Source: CAD feature listing. Evaluate the final solid. Frame: model axes, mm. A direction names the side the tool comes from. Round coordinates to 2 decimals unless told otherwise and drop trailing zeros. Loops run counter-clockwise (first coordinate to the right, second up) from the corner with the lowest first, then second, coordinate; pieces in that order, holes last. Notation, with made-up numbers: M -26,-35.5 L 28,-35.5 A30 ccw 28,-11.5 Z; hole C 86,-1 d7. An arc over 180 degrees is marked long. Answer as CSV lines item,"result". Start each with the question number.
```python
from build123d import *

# Parameters (mm, degrees)
ESBO_O3_W = 2.1
ESBO_O3_H = 15.4
FILETE1_R = 3
FILETE2_R = 0.5


with BuildPart() as part:
    # Esboço1 → Revolução1 (revolve)
    with BuildSketch(Plane.XY, mode=Mode.PRIVATE) as revolu_o1_sk:
        Polygon((0, 10.8), (0, 15.4), (15, 15.4), (15, 13.5), (50, 13.5), (50, 10.8), align=None)
    revolve(revolu_o1_sk.sketch.rotate(Axis((0, 0, 0), (1, 0, 0)), 90), axis=Axis((0, 0, 0), (1, 0, 0)))

    # Esboço3 → Furo roscado de M51 (revolve, cut)
    with BuildSketch(Plane(origin=(35, 0, 0), x_dir=(0, 0, -1), z_dir=(1, 0, 0))):
        with Locations((1.05, 7.7)):
            Rectangle(ESBO_O3_W, ESBO_O3_H)
    revolve(axis=Axis((35, -6.35, 0), (0, 1, 0)), mode=Mode.SUBTRACT)

    # Filete1
    filete1_edges = [part.edges().sort_by_distance(p)[0] for p in [
        (0, 0, -15.4),
    ]]
    fillet(filete1_edges, radius=FILETE1_R)

    # Filete2
    filete2_edges = [part.edges().sort_by_distance(p)[0] for p in [
        (50, 0, -13.5),
    ]]
    fillet(filete2_edges, radius=FILETE2_R)


solid = part.part
```
1) Contact query for flat-ended pins moving along their axis: pin 1 Ø1 at (x, z) = (37, -9) entering from +Y; pin 2 Ø1 at (x, y) = (44.5, -2.5) entering from -Z; pin 3 Ø1 at (x, y) = (41, -6.5) entering from +Z. Output: stop coordinate, or through.
2) Section C-C, the plane x = 26. Return loops of the section in (y, z).
3) Section A-A, the plane z = 0. Return loops of the section in (x, y).
4) Access query for faces 1 (the flat face through (50, -11, 2)), 2 (the cylindrical face through (32.49, 13.18, -2.93)). Directions: +Z, -Z, +X, -X, +Y, -Y. A direction counts if a zero-diameter tool reaches every point of the face in a straight line with its end or side. Return the directions, or none.
5) Mould query, pull axis Z, two halves, no side actions, for faces 3 (the cylindrical face through (34.91, 12.07, 2.1)), 4 (the cylindrical face through (9.084, 15.034, -3.338)), 5 (the flat face through (15, 14, 0)), 6 (the cylindrical face through (24.65, 6.57, -8.57)). Classes: pulls with the +Z half, pulls with the -Z half, needs draft (parallel to the pull), parting line crosses it, or undercut.
6) Ray query, line 1 along Y through (x, z) = (28, 0.5); line 2 along Y through (x, z) = (43.5, 9); line 3 along Z through (x, y) = (18.5, 7.5). Return the intervals inside material, ascending.
7) Section D-D, the plane x = 35. Return loops of the section in (y, z), and give its area (3 significant figures).
8) Section B-B, the plane y = 0. Return loops of the section in (x, z).
Findings below:
1,pin 1,"y = 10.49"
1,pin 2,"z = -13.35"
1,pin 3,"z = 12.09"
2,outline,"C 0,0 d27; hole C 0,0 d21.6"
3,outline,"M 0,-12.4 A3 ccw 3,-15.4 L 15,-15.4 L 15,-13.5 L 49.5,-13.5 A0.5 ccw 50,-13 L 50,-10.8 L 0,-10.8 Z; M 0,10.8 L 32.9,10.8 L 32.9,13.5 L 15,13.5 L 15,15.4 L 3,15.4 A3 ccw 0,12.4 Z; M 37.1,10.8 L 50,10.8 L 50,13 A0.5 ccw 49.5,13.5 L 37.1,13.5 Z"
4,face 1,"+Z, -Z, +X, +Y, -Y"
4,face 2,"+X"
5,face 3,"undercut"
5,face 4,"parting line crosses it"
5,face 5,"needs draft"
5,face 6,"undercut"
6,line 1,"-13.49 to -10.79, 10.79 to 13.49"
6,line 2,"-10.06 to -5.97, 5.97 to 10.06"
6,line 3,"-11.22 to -7.77, 7.77 to 11.22"
7,outline,"M 10.59,-2.1 A10.8 cw long 10.59,2.1 L 13.34,2.1 A13.5 ccw long 13.34,-2.1 Z"
7,area,"195 mm²"
8,outline,"M 0,-12.4 A3 ccw 3,-15.4 L 15,-15.4 L 15,-13.5 L 49.5,-13.5 A0.5 ccw 50,-13 L 50,-10.8 L 0,-10.8 Z; M 0,10.8 L 50,10.8 L 50,13 A0.5 ccw 49.5,13.5 L 15,13.5 L 15,15.4 L 3,15.4 A3 ccw 0,12.4 Z"
